Read the model definition and answer for the solid it produces. Units are mm, in the model's axes. A direction names the side the tool comes from. Round coordinates to 2 decimals unless told otherwise and drop trailing zeros. Loops run counter-clockwise (first coordinate to the right, second up) from the corner with the lowest first, then second, coordinate; pieces in that order, holes last. Notation, with made-up numbers: M -5,-9 L 2,-9 A27 cw 2,8 Z; hole C 81,43.5 d5. An arc over 180 degrees is marked long. Answer as CSV lines item,"result".
```python
from build123d import *

# Parameters (mm, degrees)
F0_W     = 77.7875
F0_H     = 47.625
F1_DEPTH = 9.525
F3_DEPTH = 9.525


with BuildPart() as f1:
    # F0 (on Top) → F1 (new body)
    with BuildSketch(Plane.XY):
        Rectangle(F0_W, F0_H)
    extrude(amount=F1_DEPTH)

    # F2 (on face) → F3 (join)
    with BuildSketch(Plane.XZ.offset(23.8125)):
        Polygon((-38.89375, 38.1), (-38.89375, 9.525), (38.89375, 9.525), (38.89375, 19.05), (-3.96875, 19.05), (-19.84375, 38.1), align=None)
    extrude(amount=-F3_DEPTH)

    # F4: F1 across plane


with BuildPart() as f1_1:
    add(f1.part)
    add(f1.part.mirror(Plane.XZ))


solid = f1_1.part
```
1) A tool of negligible diameter and unlimited length cuts with its end or side. For faces 4 (the flat face through (-9, -14.288, 21)), 5 (the flat face through (18, 19, 19.05)), 6 (the flat face through (-1, 0, 0)), from which of +Z, -Z, +X, -X, +Y, -Y can it reach the whole face along a straight path? Write none if from no direction.
Evaluation:
face 4,"+Z, +X, -X"
face 5,"+Z, +X, +Y, -Y"
face 6,"-Z, +X, -X, +Y, -Y"
2) Find section A-A, the plane z = 17. Give the vertices of the cut face in (x, y).
Evaluation:
outline,"M -38.89,-23.81 L 38.89,-23.81 L 38.89,-14.29 L -38.89,-14.29 Z; M -38.89,14.29 L 38.89,14.29 L 38.89,23.81 L -38.89,23.81 Z"
3) Find section D-D, the plane z = 32. Give the vertices of the cut face in (x, y), then the cut area to 3 significant figures.
Evaluation:
outline,"M -38.89,-23.81 L -14.76,-23.81 L -14.76,-14.29 L -38.89,-14.29 Z; M -38.89,14.29 L -14.76,14.29 L -14.76,23.81 L -38.89,23.81 Z"
area,"460 mm^2"
4) Determine the mould class of faces 1 (the flat face through (38.894, 0, 7)), 2 (the flat face through (-1, 0, 9.525)), 3 (the flat face through (-9, 23.812, 15)) for opening direction Y: released by +Y, released by -Y, zero draft, split by the parting line, or undercut.
Evaluation:
face 1,"zero draft"
face 2,"undercut"
face 3,"released by +Y"
5) Find section B-B, the plane x = -22.5. Give the vertices of the cut face in (y, z) (1 decimal).
Evaluation:
outline,"M -23.8,0 L 23.8,0 L 23.8,38.1 L 14.3,38.1 L 14.3,9.5 L -14.3,9.5 L -14.3,38.1 L -23.8,38.1 Z"
6) Straight lines are drawn through the part: line 1 (Y direction, x = 2, z = 16.5); line 2 (Z direction, x = -30, y = -5) (3 decimals); line 3 (Z direction, x = 14, y = 16). For each, find the intervals that lie inside material, in ascending order.
Evaluation:
line 1,"y = -23.81 to -14.29, 14.29 to 23.81"
line 2,"z = 0 to 9.525"
line 3,"z = 0 to 19.05"
7) Find section C-C, the plane y = 19. Give the vertices of the cut face in (x, z), then the cut area to 3 significant figures.
Evaluation:
outline,"M -38.89,0 L 38.89,0 L 38.89,19.05 L -3.97,19.05 L -19.84,38.1 L -38.89,38.1 Z"
area,"2,000 mm^2"
8) Each of these flat-tipped pins is pushed along its axis until it touches: P1, Ø7.5, axis at x = 24.5, y = 21.5, coming from the +Z side; P2, Ø2, axis at x = 23.5, y = -5.5, coming from the +Z side (3 decimals); P3, Ø4, axis at y = -18, z = 34, coming from the +X side. Where does it stop, or does it pass through?
Evaluation:
P1,"stops at z = 19.05"
P2,"stops at z = 9.525"
P3,"stops at x = -14.76"
